from build123d import *

# Parameters (mm, degrees)
SKETCH1_W           = 68.58
SKETCH1_H           = 68.58
SKETCH1_W_2         = 66
SKETCH1_H_2         = 66
BOSS_EXTRUDE1_DEPTH = 25.4
SKETCH2_W           = 101.6
SKETCH2_H           = 101.6
BOSS_EXTRUDE2_DEPTH = 6.35
SKETCH3_R           = 2.5
CUT_EXTRUDE1_DEPTH  = 7.35


with BuildPart() as part:
    # Sketch1 → Boss-Extrude1 (new body)
    with BuildSketch(Plane(origin=(0, 0, 0), x_dir=(1, 0, 0), z_dir=(0, 1, 0))):
        Rectangle(SKETCH1_W, SKETCH1_H)
        Rectangle(SKETCH1_W_2, SKETCH1_H_2, mode=Mode.SUBTRACT)
    extrude(amount=BOSS_EXTRUDE1_DEPTH)

    # Sketch2 → Boss-Extrude2 (add)
    with BuildSketch(Plane(origin=(0, 0, 0), x_dir=(1, 0, 0), z_dir=(0, 1, 0))):
        Rectangle(SKETCH2_W, SKETCH2_H)
    extrude(amount=BOSS_EXTRUDE2_DEPTH)

    # Sketch3 → Cut-Extrude1 (cut, through all)
    with BuildSketch(Plane(origin=(0, 6.35, 0), x_dir=(1, 0, 0), z_dir=(0, 1, 0))):
        with Locations((-44.45, 44.45)):
            Circle(SKETCH3_R)
        with Locations((-45.331774214, -43.550375964)):
            Circle(SKETCH3_R)
        with Locations((45.331774214, -43.550375964)):
            Circle(SKETCH3_R)
        with Locations((44.45, 44.45)):
            Circle(SKETCH3_R)
    extrude(amount=-CUT_EXTRUDE1_DEPTH, mode=Mode.SUBTRACT)


solid = part.part
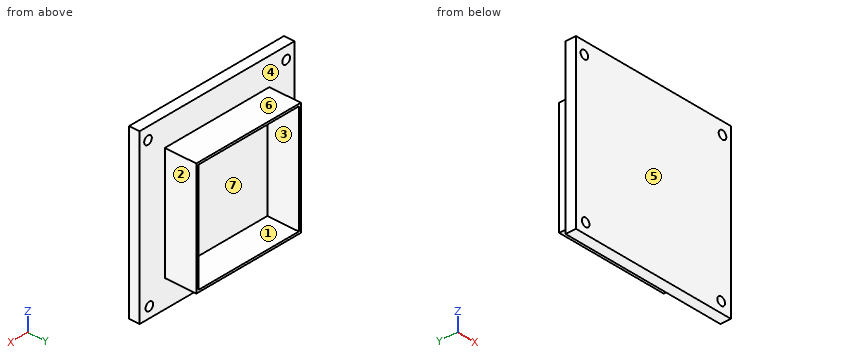
Design review of the part built by this model. Coordinates are the model's own, in mm. Face numbers are marked on the shaded views. A direction names the side the tool comes from. Round coordinates to 2 decimals unless told otherwise and drop trailing zeros. Order: outer loops, then holes, each group sorted by start corner. A loop starts at its lowest first (then second) coordinate and runs counter-clockwise, first axis right, second up.
1) Machinability: for the marked faces 5, 6 and 7, which of the approach directions +Z, -Z, +X, -X, +Y, -Y give a long, thin tool a straight path to every point of the face, cutting with its end or side? Answer none if there is none.
The answers:
face 5: +Z, -Z, +X, -X, -Y
face 6: +Z, +X, -X, +Y
face 7: +Y
2) Consider section C-C (x = -14). State the section outline as (y, z) points.
The answers:
outline: (0, -50.8) - (6.35, -50.8) - (6.35, -34.29) - (25.4, -34.29) - (25.4, -33) - (6.35, -33) - (6.35, 33) - (25.4, 33) - (25.4, 34.29) - (6.35, 34.29) - (6.35, 50.8) - (0, 50.8) - close
3) For L1, parallel to X at y = 4.75, z = -44.45; L2, parallel to X at y = 17, z = -21, list the stretches that pass through material, from the lowest coordinate up.
The answers:
L1: x = -50.8 to -46.95, -41.95 to 41.95, 46.95 to 50.8
L2: x = -34.29 to -33, 33 to 34.29
4) Clearance check with flat-ended pins moving along their axes: pin 1 Ø15 at (x, y) = (-11, 16) entering from +Z; pin 2 Ø9.5 at (x, y) = (-14.5, 18.5) entering from -Z; pin 3 Ø3 at (y, z) = (12.5, -25.5) entering from +X. State where each tip first meets the part, or that it passes through.
The answers:
pin 1: stops at z = 34.29
pin 2: stops at z = -34.29
pin 3: stops at x = 34.29
5) Consider section B-B (y = 15). State the section outline as (x, z) points, plus the area to 3 significant figures.
The answers:
outline: (-34.29, -34.29) - (34.29, -34.29) - (34.29, 34.29) - (-34.29, 34.29) - close; hole (-33, -33) - (33, -33) - (33, 33) - (-33, 33) - close
area: 347 mm2
6) Draft analysis for pull direction X (two halves, no side actions). For the marked faces 1, 2, 3 and 4, state which applies: released by +X, released by -X, zero draft, split by the parting line, or undercut.
The answers:
face 1: undercut
face 2: released by +X
face 3: undercut
face 4: zero draft
7) Consider section D-D (z = -19.5). State the section outline as (x, y) points, plus the area to 3 significant figures.
The answers:
outline: (-50.8, 0) - (50.8, 0) - (50.8, 6.35) - (34.29, 6.35) - (34.29, 25.4) - (33, 25.4) - (33, 6.35) - (-33, 6.35) - (-33, 25.4) - (-34.29, 25.4) - (-34.29, 6.35) - (-50.8, 6.35) - close
area: 694 mm2
8) Consider section A-A (z = -44.45). State the section outline as (x, y) points, plus the area to 3 significant figures.
The answers:
outline: (-50.8, 0) - (-46.95, 0) - (-46.95, 6.35) - (-50.8, 6.35) - close; (-41.95, 0) - (41.95, 0) - (41.95, 6.35) - (-41.95, 6.35) - close; (46.95, 0) - (50.8, 0) - (50.8, 6.35) - (46.95, 6.35) - close
area: 582 mm2
